Check sheet for the drawn part. Datum: minimum x, y, z corner. Units: mm. Round coordinates to 2 decimals unless told otherwise and drop trailing zeros. Write each loop counter-clockwise with the first axis right and the second up, starting at its lowest first coordinate (ties: lowest second). Pieces come first, ordered by that corner, then holes. Notation, with made-up numbers: M -16,24 L 33,24 A9 cw 33,39 Z; hole C -32.5,31 d11. An arc over 180 degrees is marked long. Put each result on its own line as item: value.
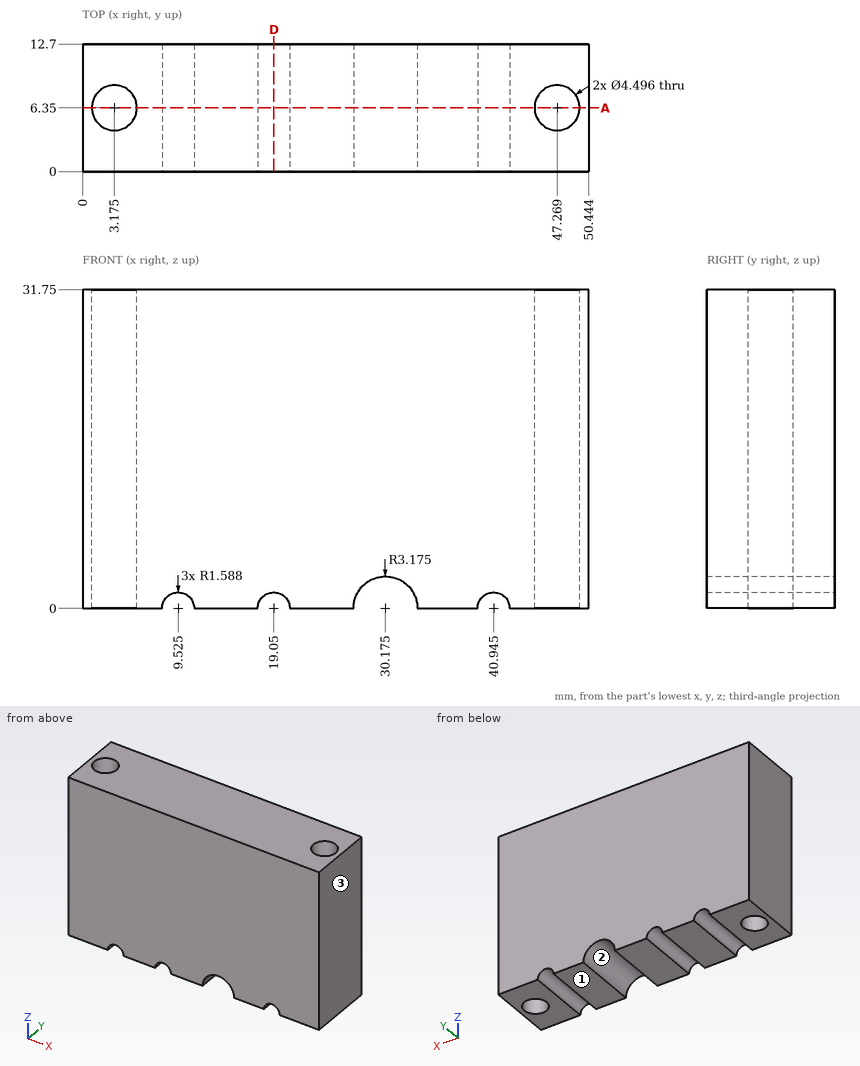
1. Cross-section at D-D (x = 19.05). Enter the section's corners in (y, z).
Computed values:
outline: M 0,1.59 L 12.7,1.59 L 12.7,31.75 L 0,31.75 Z
2. Scan lines: probe 1 along Y at (x, z) = (3, 22.5); probe 2 along X at (y, z) = (5.75, 25) (1 decimal); probe 3 along Y at (x, z) = (5, 21) (1 decimal). Record each from-to range of solid material in increasing order.
Computed values:
probe 1: y = 0 to 4.11, 8.59 to 12.7
probe 2: x = 0 to 1, 5.3 to 45.1, 49.4 to 50.4
probe 3: y = 0 to 5, 7.7 to 12.7
3. Cross-section at A-A (y = 6.35). Count the separate pieces of the cut face and the enclosed holes in it, then the cut area to 3 significant figures.
Computed values:
separate pieces: 3
enclosed holes: 0
area: 1,290 mm2
4. Release check for a two-part mould opening along X. For the marked faces 1, 2 and 3 record: +X half, -X half, draft (parallel to the pull), parting line (faces both ways), or undercut.
Computed values:
face 1: draft
face 2: undercut
face 3: +X half
5. Depth check by flat-ended pin: pin 1 Ø2.5 at (x, y) = (47.27, 6.35) entering from +Z; pin 2 Ø2 at (y, z) = (5, 28) entering from -X. Enter the tip coordinate at first touch or a pass-through.
Computed values:
pin 1: passes through
pin 2: stops at x = 0
